For this review, take the finished solid that the model builds, in its own axes (mm). Face numbers are marked on the shaded views. A direction names the side the tool comes from. Give positions to 0.01 mm unless a question says otherwise; leave off trailing zeros. Put each result on its own line as item: value. Start each with the question number.
from build123d import *

# Parameters (mm, degrees)
SKETCH3_R           = 38.22429912
SKETCH3_R_2         = 30.72429912
BOSS_EXTRUDE1_DEPTH = 25
CUT_EXTRUDE1_START  = -25
CUT_EXTRUDE1_DEPTH  = 25


with BuildPart() as part:
    # Sketch1 → Revolve1 (revolve)
    with BuildSketch(Plane.XY, mode=Mode.PRIVATE) as revolve1_sk:
        with BuildLine():
            Line((-23.22429912, -43.170194275), (-30.72429912, -43.170194275))
            Line((-30.72429912, -43.170194275), (-48.22429912, -35.38123915))
            Line((-48.22429912, -35.38123915), (-48.22429912, -11.542441336))
            Line((-48.22429912, -11.542441336), (-45.72429912, -11.542441336))
            Line((-45.72429912, -11.542441336), (-45.72429912, 41.829805725))
            Line((-45.72429912, 41.829805725), (-38.22429912, 41.829805725))
            Line((-38.22429912, 41.829805725), (-38.22429912, 16.829805725))
            Line((-38.22429912, 16.829805725), (-30.72429912, 16.829805725))
            Line((-30.72429912, 16.829805725), (-30.72429912, -29.438323417))
            ThreePointArc((-30.72429912, -29.438323417), (-28.727100264, -37.261594428), (-23.22429912, -43.170194275))
        make_face()
    revolve(revolve1_sk.sketch.rotate(Axis((0, 0, 0), (0, 1, 0)), 270), axis=Axis((0, 0, 0), (0, 1, 0)))

    # Sketch3 → Boss-Extrude1 (add)
    with BuildSketch(Plane(origin=(0, 16.829805725, 0), x_dir=(1, 0, 0), z_dir=(0, 1, 0))):
        Circle(SKETCH3_R)
        with Locations(Location((0, 0, 0), (0, 0, 90))):
            Circle(SKETCH3_R_2, mode=Mode.SUBTRACT)
    extrude(amount=BOSS_EXTRUDE1_DEPTH)

    # Sketch4 → Cut-Extrude1 (cut)
    with BuildSketch(Plane(origin=(0, 41.829805725, 0), x_dir=(1, 0, 0), z_dir=(0, 1, 0)).offset(CUT_EXTRUDE1_START)):
        with BuildLine():
            Line((-5, 37.814725075), (-5, 30.314725075))
            ThreePointArc((-5, 30.314725075), (0, 30.72429912), (5, 30.314725075))
            Line((5, 30.314725075), (5, 37.814725075))
            Line((5, 37.814725075), (-5, 37.814725075))
        make_face()
        with BuildLine():
            Line((30.254977775, -23.229071276), (23.753322024, -19.487489557))
            ThreePointArc((23.753322024, -19.487489557), (26.608023551, -15.36214956), (28.753322024, -10.827235519))
            Line((28.753322024, -10.827235519), (35.244454719, -14.587043706))
            Line((35.244454719, -14.587043706), (30.254977775, -23.229071276))
        make_face()
        with BuildLine():
            Line((-35.244454719, -14.587043706), (-28.753322024, -10.827235519))
            ThreePointArc((-28.753322024, -10.827235519), (-26.608023551, -15.36214956), (-23.753322024, -19.487489557))
            Line((-23.753322024, -19.487489557), (-30.254977775, -23.229071276))
            Line((-30.254977775, -23.229071276), (-35.244454719, -14.587043706))
        make_face()
    extrude(amount=CUT_EXTRUDE1_DEPTH, mode=Mode.SUBTRACT)


solid = part.part
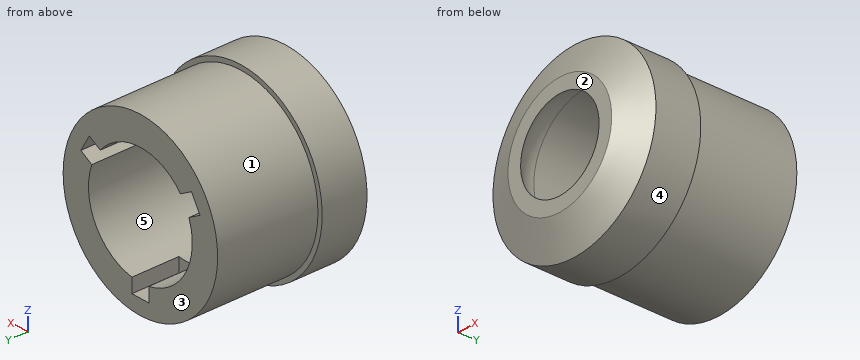
1) Wall thickness on probe 1 along X at (y, z) = (-6, 0); probe 2 along X at (y, z) = (3, -2.5); probe 3 along Z at (x, y) = (6.5, -28): over which ranges is each line inside the solid? List them lowest first.
2) Insertion check: P1, Ø8, axis at x = -1.5, y = 28, coming from the +Z side; P2, Ø3, axis at x = -30, y = -33.5, coming from the +Z side; P3, Ø5, axis at x = -34, y = 31, coming from the +Z side. Each pin has a flat end and moves straight along its axis. Give the tip position at first contact, or say it passes through.
3) Machinability: for the marked faces 1 and 2, which of the approach directions +Z, -Z, +X, -X, +Y, -Y give a long, thin tool a straight path to every point of the face, cutting with its end or side? Answer none if there is none.
4) Mouldability with a two-part tool opening along Z and no side actions: class the marked faces 3, 4 and 5 as released by +Z, released by -Z, zero draft, split by the parting line, or undercut.
Answers follow:
1. probe 1: -45.72 to -30.72, 30.72 to 45.72
1. probe 2: -45.66 to -30.62, 30.62 to 45.66
1. probe 3: -47.78 to -30.03, 30.03 to 47.78
2. P1: z = 45.72
2. P2: z = 38.9
2. P3: z = 33.14
3. face 1: +Y
3. face 2: +Z, -Z, +X, -X, -Y
4. face 3: zero draft
4. face 4: split by the parting line
4. face 5: undercut
